Verification items for the finished model (mm, model axes). A direction names the side the tool comes from. Round coordinates to 2 decimals unless told otherwise and drop trailing zeros. Order: outer loops, then holes, each group sorted by start corner. A loop starts at its lowest first (then second) coordinate and runs counter-clockwise, first axis right, second up. Notation, with made-up numbers: (74.5, 24.5) -> (93.5, 24.5) arc R32 ccw to (93.5, 52.5) -> close; hole circle Ø7 at (64.25, 24). An arc over 180 degrees is marked (long way). Put each result on its own line as item: value.
from build123d import *

# Parameters (mm, degrees)
ESQUISSE1_W              = 45.7
ESQUISSE1_H              = 28.7
BOSS_EXTRU_1_DEPTH       = 15.1
ESQUISSE2_W              = 44.1
ESQUISSE2_H              = 13.5
ENL_V_MAT_EXTRU_1_DEPTH  = 27.9
ESQUISSE3_W              = 3.040200108
ESQUISSE3_H              = 27.9
BOSS_EXTRU_2_DEPTH       = 1.3
ENL_V_MAT_EXTRU_2_DEPTH  = 1.3
ESQUISSE5_R              = 1.73665182
BOSS_EXTRU_3_DEPTH       = 1
ESQUISSE6_W              = 4.7
ESQUISSE6_H              = 1.75
ENL_V_MAT_EXTRU_3_DEPTH  = 10.5
ENL_V_MAT_EXTRU_4_DEPTH  = 10.5
BOSS_EXTRU_5_DEPTH       = 28.7
ENL_V_MAT_EXTRU_6_DEPTH  = 28.7
BOSS_EXTRU_7_DEPTH       = 3.4
ESQUISSE25_W             = 45.461360866
ESQUISSE25_H             = 0.9
ENL_V_MAT_EXTRU_14_DEPTH = 14
ENL_V_MAT_EXTRU_15_DEPTH = 57
BOSS_EXTRU_9_DEPTH       = 44.3
ESQUISSE32_R             = 0.75
ENL_V_MAT_EXTRU_17_DEPTH = 44.3
BOSS_EXTRU_10_START      = 0.5
ESQUISSE35_W             = 4.7
ESQUISSE35_H             = 1.75
BOSS_EXTRU_10_DEPTH      = 0.5
ENL_V_START              = -10
ENL_V_MAT_EXTRU_19_DEPTH = 74.3
ENL_V_START_2            = -2.2
ENL_V_MAT_EXTRU_20_DEPTH = 5
ENL_V_MAT_EXTRU_21_DEPTH = 5


with BuildPart() as part:
    # Esquisse1 → Boss.-Extru.1 (new body)
    with BuildSketch(Plane.XY):
        Rectangle(ESQUISSE1_W, ESQUISSE1_H)
    extrude(amount=BOSS_EXTRU_1_DEPTH)

    # Esquisse2 → Enlèv. mat.-Extru.1 (cut)
    with BuildSketch(Plane.XZ.offset(14.35)):
        with Locations((0, 7.8)):
            Rectangle(ESQUISSE2_W, ESQUISSE2_H)
    extrude(amount=-ENL_V_MAT_EXTRU_1_DEPTH, mode=Mode.SUBTRACT)

    # Esquisse3 → Boss.-Extru.2 (add)
    with BuildSketch(Plane.XY.offset(1.05)):
        with Locations((20.529899946, -0.4)):
            Rectangle(ESQUISSE3_W, ESQUISSE3_H)
    extrude(amount=BOSS_EXTRU_2_DEPTH)

    # Esquisse4 → Enlèv. mat.-Extru.2 (cut)
    with BuildSketch(Plane.XY.offset(15.1)):
        with BuildLine():
            Line((1.487226604, 2.215512883), (8.077709912, 2.215512883))
            Line((8.077709912, 2.215512883), (8.077709912, 2.908321808))
            Line((8.077709912, 2.908321808), (1.487226604, 2.908321808))
            ThreePointArc((1.487226604, 2.908321808), (-1.439685537, -0.018590333), (1.487226604, -2.945502474))
            Line((1.487226604, -2.945502474), (8.077709912, -2.945502474))
            Line((8.077709912, -2.945502474), (8.077709912, -2.252693548))
            Line((8.077709912, -2.252693548), (1.487226604, -2.252693548))
            ThreePointArc((1.487226604, -2.252693548), (-0.746876612, -0.018590333), (1.487226604, 2.215512883))
        make_face()
    extrude(amount=-ENL_V_MAT_EXTRU_2_DEPTH, mode=Mode.SUBTRACT)

    # Esquisse5 → Boss.-Extru.3 (add)
    with BuildSketch(Plane(origin=(0, 0, 14.55), x_dir=(-1, 0, 0), z_dir=(0, 0, -1))):
        with Locations((-1.487226604, -0.018590333)):
            Circle(ESQUISSE5_R)
    extrude(amount=BOSS_EXTRU_3_DEPTH)

    # Esquisse6 → Enlèv. mat.-Extru.3 (cut)
    with BuildSketch(Plane.XZ.offset(-13.55)):
        with Locations((2.7, 9.925)):
            Rectangle(ESQUISSE6_W, ESQUISSE6_H)
    extrude(amount=-ENL_V_MAT_EXTRU_3_DEPTH, mode=Mode.SUBTRACT)

    # Esquisse7 → Enlèv. mat.-Extru.4 (cut)
    with BuildSketch(Plane.XZ.offset(-13.55)):
        with BuildLine():
            Line((-14.95, 11.85), (-8.25, 11.85))
            ThreePointArc((-8.25, 11.85), (-6.75, 9.95), (-8.25, 8.05))
            Line((-8.25, 8.05), (-14.95, 8.05))
            ThreePointArc((-14.95, 8.05), (-16.45, 9.95), (-14.95, 11.85))
        make_face()
    extrude(amount=-ENL_V_MAT_EXTRU_4_DEPTH, mode=Mode.SUBTRACT)

    # Esquisse9 → Boss.-Extru.5 (add)
    with BuildSketch(Plane(origin=(0, 14.35, 0), x_dir=(1, 0, 0), z_dir=(0, 1, 0))):
        Polygon((22.85, 0), (22.85, -15.1), (27.85, 0), align=None)
        Polygon((-22.85, 0), (-22.85, -15.1), (-27.85, 0), align=None)
    extrude(amount=-BOSS_EXTRU_5_DEPTH)

    # Esquisse11 → Enlèv. mat.-Extru.6 (cut)
    with BuildSketch(Plane(origin=(0, 14.35, 0), x_dir=(1, 0, 0), z_dir=(0, 1, 0))):
        with BuildLine():
            Line((-25.706241432, 0), (-23.237525969, 0))
            Line((-23.237525969, 0), (-23.237525969, -0.517551291))
            Line((-23.237525969, -0.517551291), (-22.920831586, -2.2))
            ThreePointArc((-22.920831586, -2.2), (-24.475, -3.754168414), (-26.029168414, -2.2))
            Line((-26.029168414, -2.2), (-25.706241432, -0.517551291))
            Line((-25.706241432, -0.517551291), (-25.706241432, 0))
        make_face()
        with BuildLine():
            Line((23.253932079, 0), (25.706636502, 0))
            Line((25.706636502, 0), (25.706636502, -0.464338322))
            Line((25.706636502, -0.464338322), (26.030126108, -2.2))
            ThreePointArc((26.030126108, -2.2), (24.475478847, -3.754647261), (22.920831586, -2.2))
            Line((22.920831586, -2.2), (23.253932079, -0.517551291))
            Line((23.253932079, -0.517551291), (23.253932079, 0))
        make_face()
    extrude(amount=-ENL_V_MAT_EXTRU_6_DEPTH, mode=Mode.SUBTRACT)

    # Esquisse17 → Boss.-Extru.7 (add)
    with BuildSketch(Plane(origin=(0, -14.35, 0), x_dir=(-1, 0, 0), z_dir=(0, -1, 0))):
        with BuildLine():
            Line((27.85, 0), (22.85, -15.1))
            Line((22.85, -15.1), (22.05, -15.1))
            Line((22.05, -15.1), (22.05, -1.05))
            Line((22.05, -1.05), (22.05, 0))
            Line((22.05, 0), (23.237525969, 0))
            Line((23.237525969, 0), (23.237525969, -0.517551291))
            Line((23.237525969, -0.517551291), (22.920831586, -2.2))
            ThreePointArc((22.920831586, -2.2), (24.475, -3.754168414), (26.029168414, -2.2))
            Line((26.029168414, -2.2), (25.706241432, -0.517551291))
            Line((25.706241432, -0.517551291), (25.706241432, 0))
            Line((25.706241432, 0), (27.85, 0))
        make_face()
        with BuildLine():
            Line((-27.85, 0), (-22.85, -15.1))
            Line((-22.85, -15.1), (-22.055908753, -15.1))
            Line((-22.055908753, -15.1), (-22.055908753, 0))
            Line((-22.055908753, 0), (-23.253932079, 0))
            Line((-23.253932079, 0), (-23.253932079, -0.517551291))
            Line((-23.253932079, -0.517551291), (-22.920831586, -2.2))
            ThreePointArc((-22.920831586, -2.2), (-24.475478847, -3.754647261), (-26.030126108, -2.2))
            Line((-26.030126108, -2.2), (-25.706636502, -0.464338322))
            Line((-25.706636502, -0.464338322), (-25.706636502, 0))
            Line((-25.706636502, 0), (-27.85, 0))
        make_face()
    extrude(amount=BOSS_EXTRU_7_DEPTH)

    # Esquisse25 → Enlèv. mat.-Extru.14 (cut)
    with BuildSketch(Plane(origin=(0, 0, 0), x_dir=(-1, 0, 0), z_dir=(0, 0, -1))):
        with Locations((-0.047301347, -14.809065101)):
            Rectangle(ESQUISSE25_W, ESQUISSE25_H)
    extrude(amount=-ENL_V_MAT_EXTRU_14_DEPTH, mode=Mode.SUBTRACT)

    # Esquisse26 → Enlèv. mat.-Extru.15 (cut, symmetric)
    with BuildSketch(Plane(origin=(-22.05, 0, 0), x_dir=(0, 0, -1), z_dir=(1, 0, 0))):
        Polygon((-3.85, -17.75), (-15.1, -15.527418892), (-15.1, -17.75), align=None)
    extrude(amount=ENL_V_MAT_EXTRU_15_DEPTH, both=True, mode=Mode.SUBTRACT)

    # Esquisse31 → Boss.-Extru.9 (add)
    with BuildSketch(Plane.ZY.offset(-22.055908753)):
        Polygon((14.002730008, -14.35), (14.002730008, -15.744198586), (15.1, -15.527418892), (15.1, -14.35), align=None)
    extrude(amount=BOSS_EXTRU_9_DEPTH)

    # Esquisse32 → Enlèv. mat.-Extru.17 (cut)
    with BuildSketch(Plane.ZY.offset(-22.05)):
        with Locations((6.35, 1.6)):
            Circle(ESQUISSE32_R)
        with Locations((6.35, -4.4)):
            Circle(ESQUISSE32_R)
    extrude(amount=-ENL_V_MAT_EXTRU_17_DEPTH, mode=Mode.SUBTRACT)

    # Esquisse35 → Boss.-Extru.10 (add)
    with BuildSketch(Plane.XZ.offset(-13.55).offset(BOSS_EXTRU_10_START)):
        Polygon((-22.05, 14.002730008), (-22.05, 1.05), (19.009799892, 1.05), (19.009799892, 2.35), (22.05, 2.35), (22.055908753, 14.002730008), align=None)
        with Locations((2.7, 9.925)):
            Rectangle(ESQUISSE35_W, ESQUISSE35_H, mode=Mode.SUBTRACT)
        with BuildLine():
            Line((-14.95, 11.85), (-8.25, 11.85))
            ThreePointArc((-8.25, 11.85), (-6.75, 9.95), (-8.25, 8.05))
            Line((-8.25, 8.05), (-14.95, 8.05))
            ThreePointArc((-14.95, 8.05), (-16.45, 9.95), (-14.95, 11.85))
        make_face(mode=Mode.SUBTRACT)
    extrude(amount=-BOSS_EXTRU_10_DEPTH)

    # Esquisse34 → Enlèv. mat.-Extru.19 (cut)
    with BuildSketch(Plane(origin=(-22.05, 0, 0), x_dir=(0, 0, -1), z_dir=(1, 0, 0)).offset(ENL_V_START)):
        with BuildLine():
            Line((0, 11.05), (2.149848575, 13.466695377))
            Line((2.149848575, 13.466695377), (2.704974512, 17.199769042))
            Line((2.704974512, 17.199769042), (-2.5, 14.35))
            ThreePointArc((-2.5, 14.35), (-0.778882836, 13.056906943), (0, 11.05))
        make_face()
        with BuildLine():
            Line((0, -14.45), (2.615471919, -12.438405433))
            Line((2.615471919, -12.438405433), (4.64721223, -16.898892781))
            Line((4.64721223, -16.898892781), (-1.312082168, -20.336026793))
            Line((-1.312082168, -20.336026793), (-2.5, -17.75))
            ThreePointArc((-2.5, -17.75), (-0.778882836, -16.456906943), (0, -14.45))
        make_face()
    extrude(amount=ENL_V_MAT_EXTRU_19_DEPTH, mode=Mode.SUBTRACT)

    # Esquisse36 → Enlèv. mat.-Extru.20 (cut)
    with BuildSketch(Plane(origin=(-22.05, 0, 0), x_dir=(0, 0, -1), z_dir=(1, 0, 0)).offset(ENL_V_START_2)):
        with BuildLine():
            Line((-3.6, 14.35), (0.233137936, 16.139667024))
            Line((0.233137936, 16.139667024), (1.281634534, 9.28497369))
            Line((1.281634534, 9.28497369), (0, 9.85))
            ThreePointArc((0, 9.85), (-1.384829505, 12.432136396), (-3.6, 14.35))
        make_face()
        with BuildLine():
            Line((0, -13.25), (2.408593259, -12.125443566))
            Line((2.408593259, -12.125443566), (1.20429663, -19.634076372))
            Line((1.20429663, -19.634076372), (-3.6, -17.75))
            ThreePointArc((-3.6, -17.75), (-1.366017246, -15.847186204), (0, -13.25))
        make_face()
    extrude(amount=-ENL_V_MAT_EXTRU_20_DEPTH, mode=Mode.SUBTRACT)

    # Esquisse37 → Enlèv. mat.-Extru.21 (cut)
    with BuildSketch(Plane.ZY.offset(-22.05).offset(ENL_V_START_2)):
        with BuildLine():
            Line((3.6, -19.426253986), (3.6, -17.75))
            ThreePointArc((3.6, -17.75), (1.385821361, -15.831342911), (0, -13.25))
            Line((0, -13.25), (-1.954897573, -12.307105099))
            Line((-1.954897573, -12.307105099), (-2.275009075, -21.310589074))
            Line((-2.275009075, -21.310589074), (3.6, -19.426253986))
        make_face()
        with BuildLine():
            Line((3.6, 14.35), (1.25201602, 16.69798398))
            Line((1.25201602, 16.69798398), (-2.772630017, 8.353712777))
            Line((-2.772630017, 8.353712777), (0, 9.85))
            ThreePointArc((0, 9.85), (1.388075747, 12.429539402), (3.6, 14.35))
        make_face()
    extrude(amount=-ENL_V_MAT_EXTRU_21_DEPTH, mode=Mode.SUBTRACT)


solid = part.part
Item 1: Section check D-D on y = -4.4. Record the boundary of the cut face in (x, z) (3 decimals).
Check sheet entries:
outline: (-27.85, 0) -> (-25.706, 0) -> (-25.706, 0.518) -> (-26.029, 2.2) arc R1.554 cw to (-22.921, 2.2) -> (-23.238, 0.518) -> (-23.238, 0) -> (23.254, 0) -> (23.254, 0.518) -> (22.921, 2.2) arc R1.555 cw to (26.03, 2.2) -> (25.707, 0.464) -> (25.707, 0) -> (27.85, 0) -> (25.996, 5.6) -> (22.05, 5.6) -> (22.05, 2.35) -> (19.01, 2.35) -> (19.01, 1.05) -> (-22.05, 1.05) -> (-22.05, 14.55) -> (22.05, 14.55) -> (22.05, 7.1) -> (25.499, 7.1) -> (22.85, 15.1) -> (-22.85, 15.1) -> close
Item 2: Gauge pin test, flat ends, axial feed: pin 1 Ø0.6 at (y, z) = (-3.5, 0.5) entering from +X; pin 2 Ø3 at (y, z) = (2, 12) entering from -X; pin 3 Ø8 at (y, z) = (7, 8.5) entering from -X. Record the tip position at first contact, or that the pin passes through.
Check sheet entries:
pin 1: stops at x = 27.78
pin 2: stops at x = -24.37
pin 3: stops at x = -26.36
Item 3: Release check for a two-part mould opening along Z. For faces 1 (the flat face through (23.4, -17.75, 3.6)), 2 (the cylindrical face through (-0.17, 0.5, 14.06)), 3 (the flat face through (3, 14, 10.8)), 4 (the cylindrical face through (22.647, -16.481, 0.797)) record: +Z half, -Z half, draft (parallel to the pull), parting line (faces both ways), or undercut.
Check sheet entries:
face 1: draft
face 2: undercut
face 3: undercut
face 4: -Z half
Item 4: Section check C-C on x = -18.5. Record the boundary of the cut face in (y, z), then the cut area to 3 significant figures.
Check sheet entries:
outline: (-15.74, 14) -> (-14.35, 14) -> (-14.35, 14.55) -> (13.55, 14.55) -> (13.55, 14) -> (13.05, 14) -> (13.05, 1.05) -> (-14.35, 1.05) -> (-14.35, 0) -> (11.05, 0) arc R3.92 ccw to (14.35, 2.5) -> (14.35, 15.1) -> (-15.53, 15.1) -> close
area: 62.1 mm^2
Item 5: Section check A-A on y = 5.5. Record the boundary of the cut face in (x, z) (3 decimals).
Check sheet entries:
outline: (-27.85, 0) -> (-25.706, 0) -> (-25.706, 0.518) -> (-26.029, 2.2) arc R1.554 cw to (-22.921, 2.2) -> (-23.238, 0.518) -> (-23.238, 0) -> (23.254, 0) -> (23.254, 0.518) -> (22.921, 2.2) arc R1.555 cw to (26.03, 2.2) -> (25.707, 0.464) -> (25.707, 0) -> (27.85, 0) -> (22.85, 15.1) -> (-22.85, 15.1) -> close; hole (-22.05, 1.05) -> (19.01, 1.05) -> (19.01, 2.35) -> (22.05, 2.35) -> (22.05, 14.55) -> (-22.05, 14.55) -> close
Item 6: Material ranges on L1, parallel to Y at x = 23.7, z = 6.35; L2, parallel to Z at x = 10.5, y = -8; L3, parallel to X at y = -3.5, z = 1, recorded low to high. Write a range as [from, to].
Check sheet entries:
L1: y = [-17.26, -5.15], [-3.65, 0.85], [2.35, 14.35]
L2: z = [0, 1.05], [14.55, 15.1]
L3: x = [-27.52, -25.8], [-23.15, 23.16], [25.81, 27.52]
Item 7: Section check B-B on z = 6.35. State how many separate pieces and enclosed holes the cut face has, then the cut area to 3 significant figures.
Check sheet entries:
separate pieces: 3
enclosed holes: 0
area: 279 mm^2
Item 8: Tool access check on faces 5 (the flat face through (-2, -1, 1.05)), 6 (the flat face through (-0.31, -0.6, 14.55)), 7 (the flat face through (-25.87, -1.5, 1.37)). Record the directions out of +Z, -Z, +X, -X, +Y, -Y that give a thin tool (end or side, any length) a straight path to the whole face; none if there is none.
Check sheet entries:
face 5: -Y
face 6: none
face 7: +Y, -Y
